```python
from build123d import *

# Parameters (mm, degrees)
CROQUIS1_W              = 70
CROQUIS1_H              = 70
SALIENTE_EXTRUIR1_DEPTH = 70
CROQUIS2_R              = 20
SALIENTE_EXTRUIR2_DEPTH = 10
CROQUIS3_R              = 20
CORTAR_EXTRUIR1_DEPTH   = 10


with BuildPart() as part:
    # Croquis1 → Saliente-Extruir1 (new body)
    with BuildSketch(Plane.XY):
        with Locations((35, 35)):
            Rectangle(CROQUIS1_W, CROQUIS1_H)
    extrude(amount=SALIENTE_EXTRUIR1_DEPTH)

    # Croquis2 → Saliente-Extruir2 (add)
    with BuildSketch(Plane(origin=(70, 0, 0), x_dir=(0, 0, -1), z_dir=(1, 0, 0))):
        with Locations(Location((-35, 35, 0), (0, 0, 90))):
            Circle(CROQUIS2_R)
    extrude(amount=SALIENTE_EXTRUIR2_DEPTH)

    # Croquis3 → Cortar-Extruir1 (cut)
    with BuildSketch(Plane(origin=(0, 0, 0), x_dir=(-1, 0, 0), z_dir=(0, 0, -1))):
        with Locations((-35, 35)):
            Circle(CROQUIS3_R)
    extrude(amount=-CORTAR_EXTRUIR1_DEPTH, mode=Mode.SUBTRACT)


solid = part.part
```
CAD build for the part. Positions are in the model's coordinates, mm. A direction names the side the tool comes from. Give positions to 0.01 mm unless a question says otherwise; leave off trailing zeros. Order: outer loops, then holes, each group sorted by start corner. A loop starts at its lowest first (then second) coordinate and runs counter-clockwise, first axis right, second up. Notation, with made-up numbers: M 80.25,56.25 L 136.25,56.25 A16 cw 136.25,66.25 Z; hole C 84,-16.75 d1. An arc over 180 degrees is marked long. Put each result on its own line as item: value. Start each with the question number.
(1) Saw through at A-A, the plane z = 35. Write the cut outline in (x, y).
(2) Saw through at D-D, the plane z = 64. Write the cut outline in (x, y).
(3) Drill centre lines: line 1 along Y through (x, z) = (35, 4); line 2 along X through (y, z) = (9.5, 5.5); line 3 along Z through (x, y) = (38, 19.5). Where is each one in solid material? Low to high.
(4) Which spindle directions (+Z, -Z, +X, -X, +Y, -Y) get a long thin tool onto all of the face, cutting with end or side? Do faces 1 (the flat face through (35, 35, 10)), 2 (the cylindrical face through (74.93, 54.076, 41.007)), 3 (the flat face through (0, 35, 35)). Say none if no direction does.
(5) Saw through at B-B, the plane x = 35. Write the cut outline in (y, z), then the cut area to 3 significant figures.
(6) Flat gauge pins, fed straight in: pin 1 Ø6 at (x, y) = (38, 7) entering from -Z; pin 2 Ø20 at (x, y) = (42, 37.5) entering from -Z; pin 3 Ø3 at (y, z) = (61.5, 59) entering from +X. Where does each tip first touch, or does it go through?
(7) Mould opens along Y. For faces 4 (the flat face through (35, 0, 35)), 5 (the flat face through (35, 70, 35)), 6 (the flat face through (80, 35, 35)), 7 (the cylindrical face through (15.924, 41.007, 4.93)) say: +Y half, -Y half, draft (parallel to the pull), parting line (faces both ways), or undercut.
(8) Saw through at C-C, the plane y = 35. Write the cut outline in (x, z).
Check result:
1. outline: M 0,0 L 70,0 L 70,15 L 80,15 L 80,55 L 70,55 L 70,70 L 0,70 Z
2. outline: M 0,0 L 70,0 L 70,70 L 0,70 Z
3. line 1: y = 0 to 15, 55 to 70
3. line 2: x = 0 to 70
3. line 3: z = 10 to 70
4. face 1: -Z
4. face 2: +X
4. face 3: +Z, -Z, -X, +Y, -Y
5. outline: M 0,0 L 15,0 L 15,10 L 55,10 L 55,0 L 70,0 L 70,70 L 0,70 Z
5. area: 4,500 mm2
6. pin 1: stops at z = 0
6. pin 2: stops at z = 10
6. pin 3: stops at x = 70
7. face 4: -Y half
7. face 5: +Y half
7. face 6: draft
7. face 7: undercut
8. outline: M 0,0 L 15,0 L 15,10 L 55,10 L 55,0 L 70,0 L 70,15 L 80,15 L 80,55 L 70,55 L 70,70 L 0,70 Z
